from build123d import *

# Parameters (mm, degrees)
SKETCH007_W  = 28
SKETCH007_H  = 13
PAD003_DEPTH = 14.5
SKETCH008_R  = 3.3
PAD004_DEPTH = 10
PAD005_DEPTH = 16


with BuildPart() as body003:
    # Sketch007 → Pad003 (new body)
    with BuildSketch(Plane.XZ):
        with Locations((0, 2.5)):
            Rectangle(SKETCH007_W, SKETCH007_H)
    extrude(amount=PAD003_DEPTH)

    # Sketch008 (on Face6 of Pad003) → Pad004 (join)
    with BuildSketch(Plane.XZ.offset(14.5)):
        with Locations((-8, 4)):
            Circle(SKETCH008_R)
        with Locations((8, 4)):
            Circle(SKETCH008_R)
    extrude(amount=PAD004_DEPTH)


with BuildPart() as body003_1:
    # Body003 placement: moved
    add(body003.part.moved(Location((0, -16, 0))))


with BuildPart() as body004:
    # Sketch009 → Pad005 (new body)
    with BuildSketch(Plane.YZ):
        with BuildLine():
            ThreePointArc((-12, 6.4), (-16, 2.4), (-12, -1.6))
            Line((-12, -1.6), (12, -1.6))
            ThreePointArc((12, -1.6), (16, 2.4), (12, 6.4))
            Line((-12, 6.4), (12, 6.4))
        make_face()
    extrude(amount=-PAD005_DEPTH)


with BuildPart() as body004_1:
    # Body004 placement: moved
    add(body004.part.moved(Location((-22, 0, 0))))


with BuildPart() as body002:
    # Sketch006 → Revolution (revolve)
    with BuildSketch(Plane.XZ):
        Polygon((-35, -6), (-33.5, -6), (-33.5, -3), (-28, -3), (-28, 10.5), (-33.5, 10.5), (-33.5, 14), (-35, 14), align=None)
    revolve(axis=Axis((0, 0, 0), (0, 0, 1)))

    # Boolean: cut Body003
    add(body003_1.part, mode=Mode.SUBTRACT)

    # Boolean001: cut Body004
    add(body004_1.part, mode=Mode.SUBTRACT)


solid = body002.part
Geometry: final body of the model. Coordinates: model frame, mm. A direction names the side the tool comes from. Coordinates: 2 decimals unless noted, no trailing zeros. Order: outer loops, then holes, each group sorted by start corner. A loop starts at its lowest first (then second) coordinate and runs counter-clockwise, first axis right, second up. Notation, with made-up numbers: M 72.25,6 L 79.25,6 A6 cw 79.25,16 Z; hole C -11.75,52.5 d11. An arc over 180 degrees is marked long. One line per question, with ' | ' between items. Start each with the question number.
Item 1: Draft query along Z for faces 6 (the flat face through (-8, 27, 10.5)), 7 (the flat face through (0, 34, -6)), 8 (the cylindrical face through (-4.85, -32.1, 4.99)). Return one class per face: released by +Z, released by -Z, zero draft, split by the parting line, or undercut.
Item 2: Cut plane C-C, the plane y = 20.5. Return the cut outline in (x, z).
Item 3: Pin query (flat end, axial travel): pin 1 Ø1.9 at (y, z) = (-26, 2.5) entering from +X; pin 2 Ø10.5 at (x, z) = (8, 4) entering from -Y; pin 3 Ø12 at (x, y) = (-18.5, -3.5) entering from -Z (3 decimals); pin 4 Ø6.5 at (x, z) = (0, 2) entering from +Y. Return the tip coordinate at first contact, or that it passes through.
Item 4: Set-up query: faces 1 (the flat face through (-31, 0, 6.4)), 2 (the cylindrical face through (34.966, -1.539, 3.86)), 3 (the cylindrical face through (7.262, 32.703, 12.274)), 4 (the cylindrical face through (4.7, -32.1, 4.1)), 5 (the flat face through (13, 25, -3)). Return all of +Z, -Z, +X, -X, +Y, -Y with unobstructed straight access to the full face (end or side cutting, diameter ignored); none if empty.
Item 5: Cut plane B-B, the plane z = 4. Return the cut outline in (x, y), then the cut area to 3 significant figures.
Item 6: Cut plane A-A, the plane x = 0. Return the cut outline in (y, z).
Item 7: Cut plane D-D, the plane x = -8. Return the cut outline in (y, z), then the cut area to 3 significant figures.
Item 8: Ray query, probe 1 along Z at (x, y) = (-8, -31); probe 2 along Z at (x, y) = (-28, -4.5); probe 3 along Y at (x, z) = (0, 13.35). Return the intervals inside material, ascending. Write a range as [from, to].
A:
1) face 6: released by +Z | face 7: released by -Z | face 8: undercut
2) outline: M -28.37,-6 L -26.5,-6 L -26.5,-3 L -19.07,-3 L -19.07,10.5 L -26.5,10.5 L -26.5,14 L -28.37,14 Z; M 19.07,-3 L 26.5,-3 L 26.5,-6 L 28.37,-6 L 28.37,14 L 26.5,14 L 26.5,10.5 L 19.07,10.5 Z
3) pin 1: stops at x = 24.44 | pin 2: stops at y = -34.89 | pin 3: passes through | pin 4: stops at y = 35
4) face 1: -X | face 2: +Z, -Z | face 3: +Z | face 4: -Y | face 5: -Z
5) outline: M -31.3,-15.67 A35 ccw -11.3,-33.13 L -11.3,-30.5 L -14,-30.5 L -14,-24.25 A28 cw -23.21,-15.67 Z; M -31.3,15.67 L -23.21,15.67 A28 cw long 14,-24.25 L 14,-30.5 L 11.3,-30.5 L 11.3,-33.13 A35 ccw long Z; M -4.7,-34.68 A35 ccw 4.7,-34.68 L 4.7,-30.5 L -4.7,-30.5 Z | area: 1,010 mm2
6) outline: M -35,-6 L -33.5,-6 L -33.5,-3 L -30.5,-3 L -30.5,9 L -28,9 L -28,10.5 L -33.5,10.5 L -33.5,14 L -35,14 Z; M 28,-3 L 33.5,-3 L 33.5,-6 L 35,-6 L 35,14 L 33.5,14 L 33.5,10.5 L 28,10.5 Z
7) outline: M -34.07,-6 L -32.53,-6 L -32.53,-3 L -30.5,-3 L -30.5,0.7 L -34.07,0.7 Z; M -34.07,7.3 L -30.5,7.3 L -30.5,9 L -26.83,9 L -26.83,10.5 L -32.53,10.5 L -32.53,14 L -34.07,14 Z; M 26.83,-3 L 32.53,-3 L 32.53,-6 L 34.07,-6 L 34.07,14 L 32.53,14 L 32.53,10.5 L 26.83,10.5 Z | area: 148 mm2
8) probe 1: z = [-3, 0.7], [7.3, 10.5] | probe 2: z = [-3, -1.6], [6.4, 10.5] | probe 3: y = [-35, -33.5], [33.5, 35]
